Verification items for this drawing (mm, ordinates from the low corner). Give positions to 0.01 mm unless a question says otherwise; leave off trailing zeros. Loops run counter-clockwise (first coordinate to the right, second up) from the corner with the lowest first, then second, coordinate; pieces in that order, holes last. Notation, with made-up numbers: (-12, 47.5) - (44, 47.5) arc R34 ccw to (44, 84.5) - close; hole circle Ø6 at (40.5, 34.5). An arc over 180 degrees is marked (long way). One line per question, with ' | ' between items. Start each with the question number.
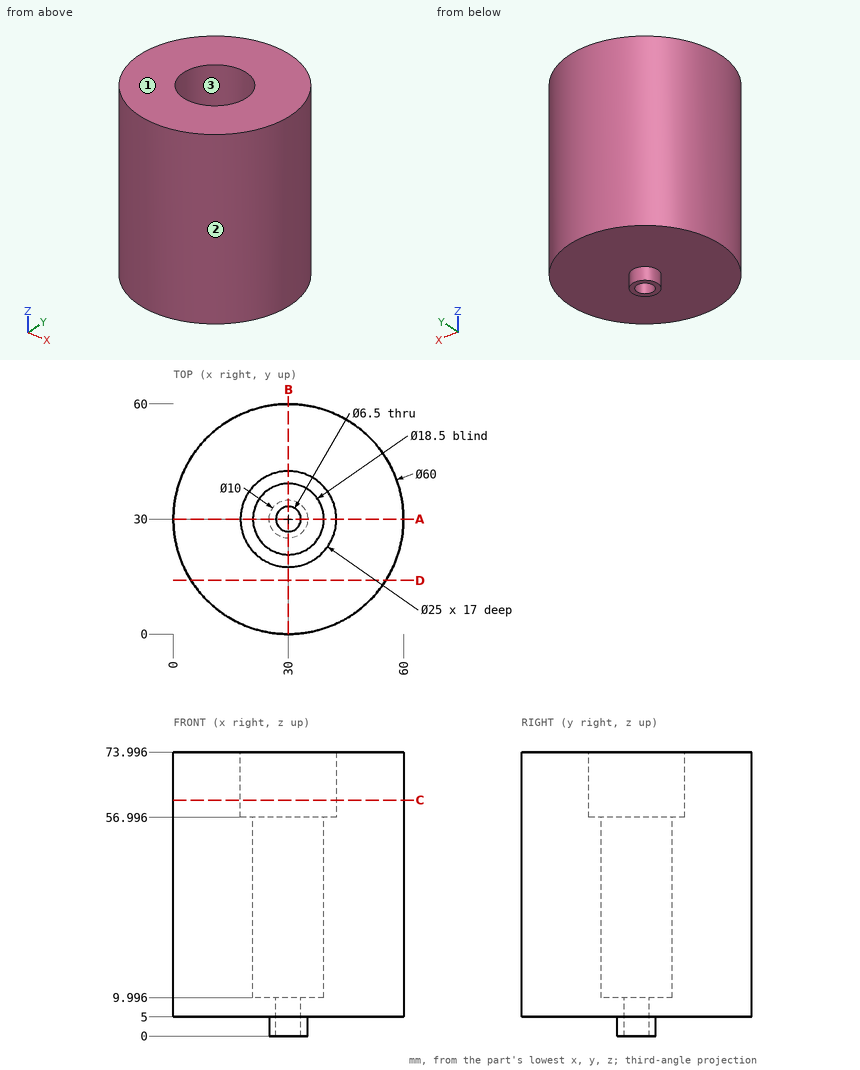
(1) Section check C-C, the plane z = 61.5. Record the boundary of the cut face in (x, y), and give its area (3 significant figures).
(2) Depth check by flat-ended pin: pin 1 Ø4 at (x, z) = (49, 64.5) entering from -Y; pin 2 Ø8 at (x, y) = (16, 22) entering from -Z; pin 3 Ø12.5 at (x, y) = (31.5, 24) entering from +Z; pin 4 Ø12 at (y, z) = (33.5, 32.5) entering from -X. Enter the tip coordinate at first touch or a pass-through.
(3) Mould release check, pull along Y, two halves, no side actions. Record for the marked faces 1, 2 and 3: pulls with the +Y half, pulls with the -Y half, needs draft (parallel to the pull), parting line crosses it, or undercut.
(4) Material ranges on line 1 (Y direction, x = 30, z = 7.75); line 2 (Z direction, x = 48, y = 15.5); line 3 (Z direction, x = 27.5, y = 24.5), recorded low to high.
(5) Section check A-A, the plane y = 30. Record the boundary of the cut face in (x, z).
(6) Section check D-D, the plane y = 14. Record the boundary of the cut face in (x, z).
Numbers:
1) outline: circle Ø60 at (30, 30); hole circle Ø25 at (30, 30) | area: 2,340 mm^2
2) pin 1: y = 5.28 | pin 2: z = 5 | pin 3: z = 57 | pin 4: x = 0
3) face 1: needs draft | face 2: parting line crosses it | face 3: undercut
4) line 1: 0 to 26.75, 33.25 to 60 | line 2: 5 to 74 | line 3: 5 to 10
5) outline: (0, 5) - (25, 5) - (25, 0) - (26.75, 0) - (26.75, 10) - (20.75, 10) - (20.75, 57) - (17.5, 57) - (17.5, 74) - (0, 74) - close; (33.25, 0) - (35, 0) - (35, 5) - (60, 5) - (60, 74) - (42.5, 74) - (42.5, 57) - (39.25, 57) - (39.25, 10) - (33.25, 10) - close
6) outline: (4.62, 5) - (55.38, 5) - (55.38, 74) - (4.62, 74) - close
